```python
from build123d import *

# Parameters (mm, degrees)
F0_W     = 1270
F0_H     = 635
F0_W_2   = 1219.2
F0_H_2   = 609.6
F1_DEPTH = 635
F2_DEPTH = 609.6
F3_R     = 25.4
F3_R_2   = 12.7
F4_DEPTH = 50.8


with BuildPart() as f1:
    # F0 (on Front) → F1 (new body)
    with BuildSketch(Plane.XZ):
        Rectangle(F0_W, F0_H)
        Rectangle(F0_W_2, F0_H_2, mode=Mode.SUBTRACT)
        Rectangle(F0_W_2, F0_H_2)
    extrude(amount=F1_DEPTH)

    # F0 (on Front) → F2 (cut)
    with BuildSketch(Plane.XZ):
        Rectangle(F0_W_2, F0_H_2)
    extrude(amount=F2_DEPTH, mode=Mode.SUBTRACT)

    # F3 (on face) → F4 (join)
    with BuildSketch(Plane(origin=(0, 0, -317.5), x_dir=(1, 0, 0), z_dir=(0, 0, -1))):
        with Locations((317.5, 317.5)):
            Circle(F3_R)
        with Locations((317.5, 317.5)):
            Circle(F3_R_2, mode=Mode.SUBTRACT)
        with Locations((-317.5, 317.5)):
            Circle(F3_R)
        with Locations((-317.5, 317.5)):
            Circle(F3_R_2, mode=Mode.SUBTRACT)
    extrude(amount=F4_DEPTH)


solid = f1.part
```
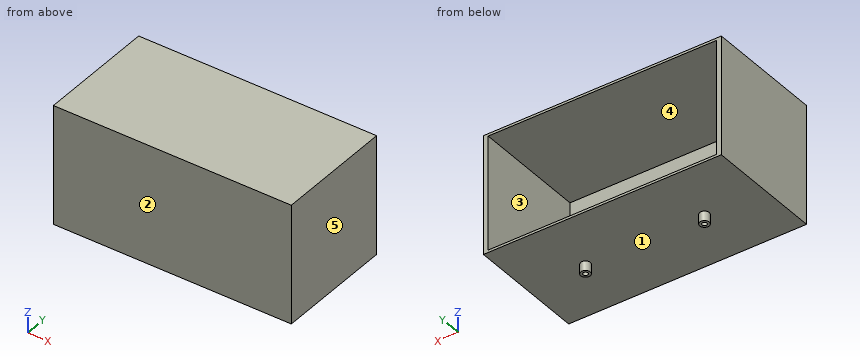
Build history of the part. All positions in model axes, mm. Face numbers are marked on the shaded views. A direction names the side the tool comes from. Give positions to 0.01 mm unless a question says otherwise; leave off trailing zeros. Order: outer loops, then holes, each group sorted by start corner. A loop starts at its lowest first (then second) coordinate and runs counter-clockwise, first axis right, second up. Notation, with made-up numbers: M 26.25,84.25 L 47.25,84.25 A27 cw 47.25,109.25 Z; hole C 17,17 d10. An arc over 180 degrees is marked long. Write item = value, one per line. Start each with the question number.
(1) Slice it at B-B on x = -425.5. Write the cut outline in (y, z), plus the area to 3 significant figures.
(2) Probe L1, parallel to X at y = -317.5, z = -329; L2, parallel to Z at x = 158, y = -366; L3, parallel to X at y = -456, z = 208. List the from-to ranges inside material, lowest first. Write a range as [from, to].
(3) Which spindle directions (+Z, -Z, +X, -X, +Y, -Y) get a long thin tool onto all of the face, cutting with end or side? Do the marked faces 4 and 5. Say none if no direction does.
(4) Slice it at C-C on z = 133.5. Write the cut outline in (x, y), plus the area to 3 significant figures.
(5) Pin check, flat tips, straight feed: pin 1 Ø12 at (x, y) = (405.5, -533.5) entering from -Z; pin 2 Ø20.5 at (x, y) = (-314, -315.5) entering from -Z; pin 3 Ø4 at (x, z) = (288, -75) entering from +Y. Stop position of each tip, or through.
(6) Slice it at D-D on y = -317.5. Write the cut outline in (x, z).
(7) Slice it at A-A on y = -437. Write the cut outline in (x, z).
(8) Two-plate mould, pull along Z, no slides. Class the marked faces 1, 2 and 3: released by +Z, released by -Z, zero draft, split by the parting line, or undercut.
Responses:
q1.outline = M -635,-317.5 L 0,-317.5 L 0,-304.8 L -609.6,-304.8 L -609.6,304.8 L 0,304.8 L 0,317.5 L -635,317.5 Z
q1.area = 31,600 mm2
q2.L1 = [-342.9, -330.2], [-304.8, -292.1], [292.1, 304.8], [330.2, 342.9]
q2.L2 = [-317.5, -304.8], [304.8, 317.5]
q2.L3 = [-635, -609.6], [609.6, 635]
q3.face_4 = +Y
q3.face_5 = +Z, -Z, +X, +Y, -Y
q4.outline = M -635,-635 L 635,-635 L 635,0 L 609.6,0 L 609.6,-609.6 L -609.6,-609.6 L -609.6,0 L -635,0 Z
q4.area = 63,200 mm2
q5.pin_1 = -317.5
q5.pin_2 = -368.3
q5.pin_3 = -609.6
q6.outline = M -635,-317.5 L -342.9,-317.5 L -342.9,-368.3 L -330.2,-368.3 L -330.2,-317.5 L -304.8,-317.5 L -304.8,-368.3 L -292.1,-368.3 L -292.1,-317.5 L 292.1,-317.5 L 292.1,-368.3 L 304.8,-368.3 L 304.8,-317.5 L 330.2,-317.5 L 330.2,-368.3 L 342.9,-368.3 L 342.9,-317.5 L 635,-317.5 L 635,317.5 L -635,317.5 Z; hole M -609.6,-304.8 L 609.6,-304.8 L 609.6,304.8 L -609.6,304.8 Z
q7.outline = M -635,-317.5 L 635,-317.5 L 635,317.5 L -635,317.5 Z; hole M -609.6,-304.8 L 609.6,-304.8 L 609.6,304.8 L -609.6,304.8 Z
q8.face_1 = released by -Z
q8.face_2 = zero draft
q8.face_3 = undercut
